Read the model definition and answer for the solid it produces. Units are mm, in the model's axes. A direction names the side the tool comes from. Give positions to 0.01 mm unless a question says otherwise; leave off trailing zeros. Order: outer loops, then holes, each group sorted by start corner. A loop starts at its lowest first (then second) coordinate and runs counter-clockwise, first axis right, second up. Notation, with made-up numbers: (29.5, -29.75) -> (40.5, -29.75) arc R19 ccw to (40.5, -24.75) -> close; hole circle Ø10 at (78.5, -40). An arc over 180 degrees is marked (long way). Answer as CSV lines item,"result". Start each with the question number.
1) The mould has two halves that part along Y. Classify faces 1 (the face through (25, -251, 80)), 2 (the face through (25, -694, 100)), 3 (the face through (25, 0, 51)): +Y half, -Y half, draft (parallel to the pull), parting line (faces both ways), or undercut.
2) Find section B-B (y = -230). Determine the outline of the cut face in (x, z), and give its area (3 significant figures).
3) Flat-ended cylindrical pins translate along their axes: pin 1 Ø22 at (x, z) = (25.5, 90) entering from +Y; pin 2 Ø15 at (x, y) = (33, -1126.5) entering from +Z. Find the tip coordinate at first contact, or state that the pin passes through.
4) For faces 4 (the face through (25, -690, 0)), 5 (the face through (25, -1151, 80)), determine the directions among +Z, -Z, +X, -X, +Y, -Y from which every point of the face is accessible in a straight line to the end or side of a thin tool.
5) Find section A-A (x = 31.5). Determine the outline of the cut face in (y, z), and give its area (3 significant figures).
6) Straight lines are drawn through the part: L1, parallel to Y at x = 33.5, z = 85.5; L2, parallel to Z at x = 26, y = -298. For each, find the intervals that lie inside material, in ascending order. Write a range as from..to.
```python
from build123d import *

# Parameters (mm, degrees)
F0_W     = 50
F0_H     = 100
F1_DEPTH = 1400
F2_W     = 100
F2_H     = 20
F3_DEPTH = 50.001


with BuildPart() as f1:
    # F0 (on Front) → F1 (new body)
    with BuildSketch(Plane.XZ):
        with Locations((25, 50)):
            Rectangle(F0_W, F0_H)
    extrude(amount=F1_DEPTH)

    # F2 (on face) → F3 (cut, through all)
    with BuildSketch(Plane.YZ.offset(50)):
        with Locations((-250, 90)):
            Rectangle(F2_W, F2_H)
        with Locations((-1150, 90)):
            Rectangle(F2_W, F2_H)
    extrude(amount=-F3_DEPTH, mode=Mode.SUBTRACT)


solid = f1.part
```
Findings below:
1,face 1,"undercut"
1,face 2,"draft"
1,face 3,"+Y half"
2,outline,"(0, 0) -> (50, 0) -> (50, 80) -> (0, 80) -> close"
2,area,"4,000 mm²"
3,pin 1,"y = 0"
3,pin 2,"z = 80"
4,face 4,"-Z, +X, -X, +Y, -Y"
4,face 5,"+Z, +X, -X"
5,outline,"(-1400, 0) -> (0, 0) -> (0, 100) -> (-200, 100) -> (-200, 80) -> (-300, 80) -> (-300, 100) -> (-1100, 100) -> (-1100, 80) -> (-1200, 80) -> (-1200, 100) -> (-1400, 100) -> close"
5,area,"136,000 mm²"
6,L1,"-1400..-1200, -1100..-300, -200..0"
6,L2,"0..80"
